Can you work these out from the drawing? Everything is in mm from the part's minimum corner. A direction names the side the tool comes from. Coordinates: 2 decimals unless noted, no trailing zeros. Loops run counter-clockwise (first coordinate to the right, second up) from the corner with the lowest first, then second, coordinate; pieces in that order, holes last. Notation, with made-up numbers: (0.25, 16) - (51.25, 16) arc R26 cw to (51.25, 54) - close; hole circle Ø2 at (86, 88.5). An arc over 180 degrees is marked (long way). One line per question, with ' | ' between items. Start each with the question number.
1. Which directions (+Z, -Z, +X, -X, +Y, -Y) give clear straight access to the entire face, cutting with the end or side of a thin tool? Please do the marked faces 1 and 2.
2. I'm going to push flat-ended pins straight in: P1, Ø10, axis at x = 105.5, y = 56.5, coming from the +Z side; P2, Ø1.5, axis at y = 75.5, z = 17.5, coming from the +X side. Where does each tip first touch, or does it pass through?
3. Please list where these lines run through material, in increasing order: L1, parallel to X at y = 67, z = 13; L2, parallel to Y at x = 125, z = 43.5; L3, parallel to X at y = 69.5, z = 17. Write a range as [from, to].
4. We'd pull the mould along X, two halves only. Please class the marked faces 3, 4 and 5: pulls with the +X half, pulls with the -X half, needs draft (parallel to the pull), parting line crosses it, or undercut.
5. I want a section at C-C, the plane y = 43.5. Write out the boundary of the cut face in (x, z), then the cut area to 3 significant figures.
6. I want a section at A-A, the plane z = 38.5. Write out the boundary of the cut face in (x, y), then the cut area to 3 significant figures.
7. I want a section at D-D, the plane y = 6. Write out the boundary of the cut face in (x, z), then the cut area to 3 significant figures.
8. I want a section at B-B, the plane x = 114.5. Write out the boundary of the cut face in (y, z).
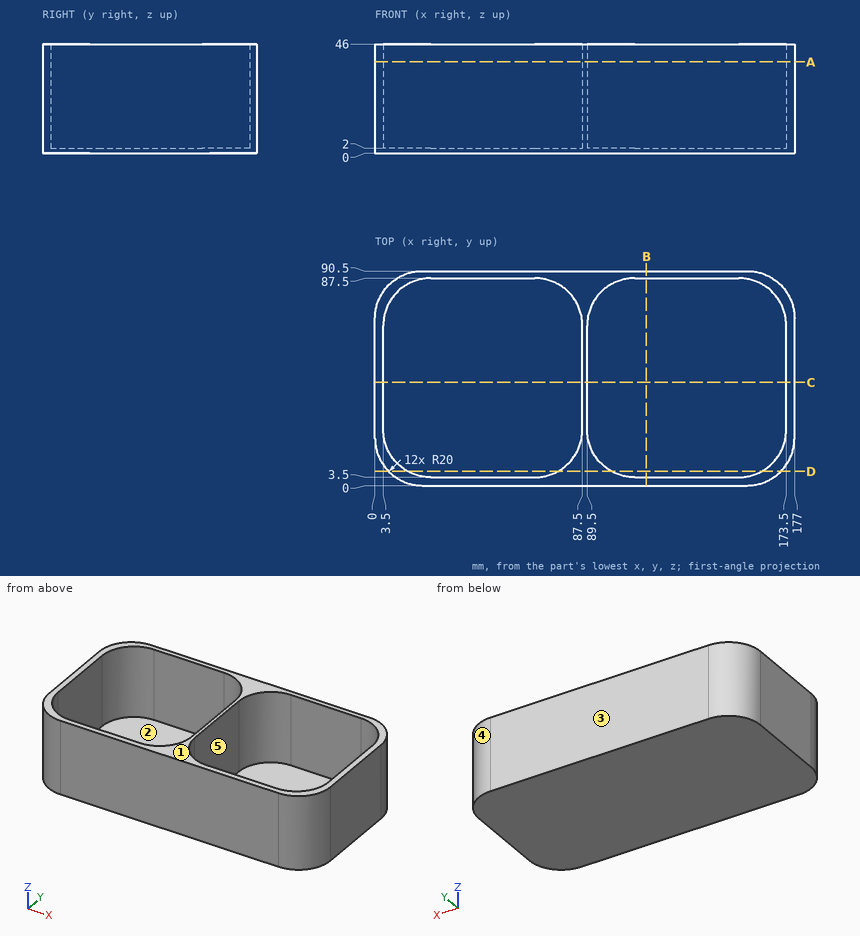
Results are:
1) face 1: +Z, +X, -X, +Y, -Y | face 2: +Z
2) P1: stops at z = 2 | P2: stops at x = 176.54
3) L1: x = [0, 3.5], [87.5, 89.5], [173.5, 177] | L2: y = [0, 3.5], [87.5, 90.5] | L3: x = [0, 3.6], [87.4, 89.6], [173.4, 177]
4) face 3: needs draft | face 4: pulls with the +X half | face 5: undercut
5) outline: (0, 0) - (177, 0) - (177, 46) - (173.5, 46) - (173.5, 2) - (89.5, 2) - (89.5, 46) - (87.5, 46) - (87.5, 2) - (3.5, 2) - (3.5, 46) - (0, 46) - close | area: 750 mm2
6) outline: (0, 20) arc R20 ccw to (20, 0) - (157, 0) arc R20 ccw to (177, 20) - (177, 70.5) arc R20 ccw to (157, 90.5) - (20, 90.5) arc R20 ccw to (0, 70.5) - close; hole (3.5, 23.5) arc R20 ccw to (23.5, 3.5) - (67.5, 3.5) arc R20 ccw to (87.5, 23.5) - (87.5, 67.5) arc R20 ccw to (67.5, 87.5) - (23.5, 87.5) arc R20 ccw to (3.5, 67.5) - close; hole (89.5, 23.5) arc R20 ccw to (109.5, 3.5) - (153.5, 3.5) arc R20 ccw to (173.5, 23.5) - (173.5, 67.5) arc R20 ccw to (153.5, 87.5) - (109.5, 87.5) arc R20 ccw to (89.5, 67.5) - close | area: 2,250 mm2
7) outline: (5.72, 0) - (171.28, 0) - (171.28, 46) - (163.18, 46) - (163.18, 2) - (99.82, 2) - (99.82, 46) - (77.18, 46) - (77.18, 2) - (13.82, 2) - (13.82, 46) - (5.72, 46) - close | area: 2,040 mm2
8) outline: (0, 0) - (90.5, 0) - (90.5, 46) - (87.5, 46) - (87.5, 2) - (3.5, 2) - (3.5, 46) - (0, 46) - close
